Geometry check sheet. Reference: the model listing, model coordinates, mm. A direction names the side the tool comes from. Round coordinates to 2 decimals unless told otherwise and drop trailing zeros. Loops run counter-clockwise (first coordinate to the right, second up) from the corner with the lowest first, then second, coordinate; pieces in that order, holes last. Notation, with made-up numbers: M 11,86 L 22,86 A11 ccw 22,90 Z; hole C 4,21 d5. An arc over 180 degrees is marked long. Use one line per item in the form item = value. Start each with the question number.
1. Cross-section at A-A (x = 12). Record the boundary of the cut face in (y, z), then the cut area to 3 significant figures.
2. Set-up check for faces 1 (the flat face through (0, 89, 7.388)), 2 (the flat face through (19.05, -851, 43)), 3 (the flat face through (0, -1714.673, -3)), 4 (the flat face through (0, 89, 58.188)), 5 (the flat face through (0, -1766, 67.072)): record each of +Z, -Z, +X, -X, +Y, -Y from which the full face is reachable in a straight line by a thin tool's end or side.
3. Go/stop test with flat-tipped pins: pin 1 (4 mm diameter, centred on x = 13.5, z = 80, fed in from -Y); pin 2 (19 mm diameter, centred on x = 5, y = 109.5, fed in from -Z). Record where each tip stops, or that it passes through.
4. Material ranges on line 1 (Y direction, x = 10, z = 3); line 2 (Y direction, x = -15, z = 0); line 3 (Z direction, x = -7.5, y = 48), recorded low to high.
5. Cross-section at B-B (z = 83). Record the boundary of the cut face in (x, y).
```python
from build123d import *

# Parameters (mm, degrees)
F1_DEPTH = 19.05
F0_W     = 101.6
F0_H     = 50.8
F2_DEPTH = 19.05


with BuildPart() as f1:
    # F0 (on Right) → F1 (new body, symmetric)
    with BuildSketch(Plane.YZ):
        Polygon((-1714.672583, 105.171546), (-1714.672583, 67.071546), (-1714.672583, 16.271546), (-1714.672583, -21.828454), (37.927417, -21.828454), (39.198343, 7.38804), (39.198343, 58.18804), (37.927417, 105.171546), align=None)
    extrude(amount=F1_DEPTH, both=True)

    # F0 (on Right) → F2 (join, symmetric)
    with BuildSketch(Plane.YZ):
        with Locations((89.998343, 32.78804)):
            Rectangle(F0_W, F0_H)
        with Locations((-1765.472583, 41.671546)):
            Rectangle(F0_W, F0_H)
    extrude(amount=F2_DEPTH, both=True)


solid = f1.part
```
Reported:
q1.outline = M -1816.27,16.27 L -1714.67,16.27 L -1714.67,-21.83 L 37.93,-21.83 L 39.2,7.39 L 140.8,7.39 L 140.8,58.19 L 39.2,58.19 L 37.93,105.17 L -1714.67,105.17 L -1714.67,67.07 L -1816.27,67.07 Z
q1.area = 233,000 mm²
q2.face_1 = -Z, +X, -X, +Y
q2.face_2 = +Z, -Z, +X, +Y, -Y
q2.face_3 = -Z, +X, -X, -Y
q2.face_4 = +Z, +X, -X, +Y
q2.face_5 = +Z, +X, -X, -Y
q3.pin_1 = -1714.67
q3.pin_2 = 7.39
q4.line_1 = -1714.67 to 39.01
q4.line_2 = -1714.67 to 38.88
q4.line_3 = 7.39 to 58.19
q5.outline = M -19.05,-1714.67 L 19.05,-1714.67 L 19.05,38.53 L -19.05,38.53 Z
